Part model, mm, in its own coordinate system. Coordinates: 2 decimals unless noted, no trailing zeros. Loops run counter-clockwise (first coordinate to the right, second up) from the corner with the lowest first, then second, coordinate; pieces in that order, holes last. Notation, with made-up numbers: M 64.5,84 L 69.5,84 A8 cw 69.5,88 Z; hole C 15.25,79 d7. An arc over 180 degrees is marked long. Use a Markdown table: item, result. Add a question column.
1) Pull direction Z, two halves, no side cores. Call faces 1 (the flat face through (65.353, -0.021, 79.495)), 2 (the cylindrical face through (141.34, 0.02, 142.11)), 3 (the cylindrical face through (-38.355, 0.021, 0.11)), 4 (the flat face through (74.606, -0.021, 60.464)): released by +Z, released by -Z, zero draft, split by the parting line, or undercut.
2) Wall check: probe 1 along Z at (x, y) = (70, 0.4); probe 2 along Z at (x, y) = (-24.5, 0.15); probe 3 along X at (y, z) = (0.2, 140). Give the ranges that are in metal, low to high. Write a range as from..to.
3) Band-saw the part on D-D (x = -11.5). List the corners of the cut face in (y, z), plus the area to 3 significant figures.
4) Band-saw the part on A-A (y = 0.35). List the corners of the cut face in (x, z), plus the area to 3 significant figures.
5) Band-saw the part on C-C (z = 70). List the corners of the cut face in (x, y), plus the area to 3 significant figures.
6) Band-saw the part on B-B (x = 70). List the corners of the cut face in (y, z), plus the area to 3 significant figures.
7) Pin check, flat tips, straight feed: pin 1 Ø4 at (x, z) = (70, 70) entering from +Y; pin 2 Ø1.5 at (x, y) = (34, 0.5) entering from -Z; pin 3 Ø1.5 at (y, z) = (0.5, -14.5) entering from -X; pin 4 Ø0.9 at (x, y) = (-29, 0) entering from -Z. Stop position of each tip, or through.
from build123d import *

# Parameters (mm, degrees)
F0_R     = 2.5
F1_DEPTH = 1.5


with BuildPart() as f1:
    # F0 (on Front) → F1 (new body, symmetric)
    with BuildSketch(Plane.XZ):
        with BuildLine():
            Line((-4.142136, 10), (-35.857864, 10))
            ThreePointArc((-35.857864, 10), (-45.857864, 0), (-35.857864, -10))
            Line((-35.857864, -10), (-15.857864, -10))
            Line((-15.857864, -10), (-15.857864, -25))
            Line((-15.857864, -25), (4.142136, -25))
            Line((4.142136, -25), (4.142136, -10))
            Line((4.142136, -10), (147.071068, 132.928932))
            ThreePointArc((147.071068, 132.928932), (147.071068, 147.071068), (132.928932, 147.071068))
            Line((132.928932, 147.071068), (-4.142136, 10))
        make_face()
        with Locations((-35.857864, 0)):
            Circle(F0_R, mode=Mode.SUBTRACT)
        with Locations((70, 70)):
            Circle(F0_R, mode=Mode.SUBTRACT)
        with Locations((140, 140)):
            Circle(F0_R, mode=Mode.SUBTRACT)
    extrude(amount=F1_DEPTH, both=True)


solid = f1.part
Entries:
| question | item | result |
|---|---|---|
| 1 | face 1 | released by +Z |
| 1 | face 2 | undercut |
| 1 | face 3 | undercut |
| 1 | face 4 | released by -Z |
| 2 | probe 1 | 55.86..67.5, 72.5..84.14 |
| 2 | probe 2 | -10..10 |
| 2 | probe 3 | 125.86..137.5, 142.5..150 |
| 3 | outline | M -1.5,-25 L 1.5,-25 L 1.5,10 L -1.5,10 Z |
| 3 | area | 105 mm2 |
| 4 | outline | M -35.86,-10 L -15.86,-10 L -15.86,-25 L 4.14,-25 L 4.14,-10 L 147.07,132.93 A10 ccw 132.93,147.07 L -4.14,10 L -35.86,10 A10 ccw Z; hole C -35.86,0 d5; hole C 70,70 d5; hole C 140,140 d5 |
| 4 | area | 5,230 mm2 |
| 5 | outline | M 55.86,-1.5 L 67.5,-1.5 L 67.5,1.5 L 55.86,1.5 Z; M 72.5,-1.5 L 84.14,-1.5 L 84.14,1.5 L 72.5,1.5 Z |
| 5 | area | 69.9 mm2 |
| 6 | outline | M -1.5,55.86 L 1.5,55.86 L 1.5,67.5 L -1.5,67.5 Z; M -1.5,72.5 L 1.5,72.5 L 1.5,84.14 L -1.5,84.14 Z |
| 6 | area | 69.9 mm2 |
| 7 | pin 1 | through |
| 7 | pin 2 | z = 19.11 |
| 7 | pin 3 | x = -15.86 |
| 7 | pin 4 | z = -10 |
